```python
from build123d import *
from build123d.topology import SkipClean

# Parameters (mm, degrees)
BOSS_EXTRUDE1_DEPTH      = 10
SKETCH4_R                = 1.962636903
CUT_EXTRUDE2_DEPTH       = 10
SKETCH6_R                = 2.5
SKETCH6_R_2              = 1.962636903
BOSS_EXTRUDE2_DEPTH      = 3.333333333
BOSS_EXTRUDE3_START      = -3.333333333
SKETCH7_R                = 2.5
SKETCH7_R_2              = 1.962636903
BOSS_EXTRUDE3_DEPTH      = 3.333333333
SKETCH9_W                = 3.333333334
SKETCH9_H                = 5
CUT_EXTRUDE7_DEPTH       = 3
SKETCH10_W               = 3.333333334
SKETCH10_H               = 1.037363097
CUT_EXTRUDE8_DEPTH       = 37.201372358
BOSS_EXTRUDE4_DEPTH      = 1.5
BOSS_EXTRUDE4_DEPTH_BACK = 1.5
SKETCH12_R               = 2
BOSS_EXTRUDE9_DEPTH      = 1.5
BOSS_EXTRUDE9_DEPTH_BACK = 1.5
CUT_EXTRUDE9_DEPTH       = 40.05524944


with BuildPart() as part:
    # Sketch3 → Boss-Extrude1 (new body)
    with BuildSketch(Plane(origin=(0, 0, 0), x_dir=(0, 0, -1), z_dir=(1, 0, 0))):
        Polygon((30, 2.5), (31.962636903, 2.5), (31.97894003, 5), (30, 5), (0, 5), (0, 0), (30, 0), align=None)
    extrude(amount=BOSS_EXTRUDE1_DEPTH)

    # Sketch4 → Cut-Extrude2 (cut)
    with BuildSketch(Plane(origin=(0, 0, 0), x_dir=(0, 0, -1), z_dir=(1, 0, 0))):
        with Locations((31.962636903, 2.5)):
            Circle(SKETCH4_R)
    extrude(amount=CUT_EXTRUDE2_DEPTH, mode=Mode.SUBTRACT)

    # Sketch6 → Boss-Extrude2 (add)
    with BuildSketch(Plane.ZY):
        with Locations((-31.962636903, 2.5)):
            Circle(SKETCH6_R)
        with Locations((-31.962636903, 2.5)):
            Circle(SKETCH6_R_2, mode=Mode.SUBTRACT)
    extrude(amount=-BOSS_EXTRUDE2_DEPTH)

    # Sketch7 → Boss-Extrude3 (add)
    with BuildSketch(Plane(origin=(10, 0, 0), x_dir=(0, 0, -1), z_dir=(1, 0, 0)).offset(BOSS_EXTRUDE3_START)):
        with Locations((31.962636903, 2.5)):
            Circle(SKETCH7_R)
        with Locations((31.962636903, 2.5)):
            Circle(SKETCH7_R_2, mode=Mode.SUBTRACT)
    extrude(amount=BOSS_EXTRUDE3_DEPTH)

    # Sketch9 → Cut-Extrude7 (cut)
    with SkipClean():  # the faces are left unmerged after this step: merging them gives an invalid solid
        with BuildSketch(Plane(origin=(0, -0.208321197, -31.944975261), x_dir=(-1, 0, 0), z_dir=(0, -0.006521112201233067, -0.9999787373217788))):
            with Locations((-5, 2.708378785)):
                Rectangle(SKETCH9_W, SKETCH9_H)
        extrude(amount=-CUT_EXTRUDE7_DEPTH, mode=Mode.SUBTRACT)

    # Sketch10 → Cut-Extrude8 (cut, through all)
    with SkipClean():  # the faces are left unmerged after this step: merging them gives an invalid solid
        with BuildSketch(Plane(origin=(0, 0.208374354, -0.001358861), x_dir=(1, 0, 0), z_dir=(0, 0.9999787373217788, -0.00652111220123307))):
            with Locations((5, 29.464336059)):
                Rectangle(SKETCH10_W, SKETCH10_H)
        extrude(amount=-CUT_EXTRUDE8_DEPTH, mode=Mode.SUBTRACT)

    # Sketch12 → Boss-Extrude4 (add, two sides: drawn at the far end of the back side and taken through both)
    with SkipClean():  # the faces are left unmerged after this step: merging them gives an invalid solid
        with BuildSketch(Plane(origin=(5, 0, 0), x_dir=(0, 0, -1), z_dir=(1, 0, 0)).offset(-BOSS_EXTRUDE4_DEPTH_BACK)):
            with BuildLine():
                Line((-2.5, 5), (0, 5))
                Line((0, 5), (0, 2.5))
                ThreePointArc((0, 2.5), (-4.267766953, 0.732233047), (-2.5, 5))
            make_face()
            with Locations((-2.5, 2.5)):
                Circle(SKETCH12_R, mode=Mode.SUBTRACT)
        extrude(amount=BOSS_EXTRUDE4_DEPTH + BOSS_EXTRUDE4_DEPTH_BACK)

    # Sketch13 → Boss-Extrude9 (add, two sides: drawn at the far end of the back side and taken through both)
    with SkipClean():  # the faces are left unmerged after this step: merging them gives an invalid solid
        with BuildSketch(Plane(origin=(5, 0, 0), x_dir=(0, 0, -1), z_dir=(1, 0, 0)).offset(-BOSS_EXTRUDE9_DEPTH_BACK)):
            with BuildLine():
                Line((24.809137755, 5), (28, 5))
                Line((28, 5), (38, 5))
                Line((38, 5), (38, 6.25))
                Line((38, 6.25), (28, 6.25))
                add(Edge.make_bspline(
                    [(28, 6.25), (27.570139782, 6.25), (27.108034748, 5.787413316), (26.444737385, 5.323894947), (26.11400028, 5.04700236), (24.809137755, 5.04700236)],
                    knots=[0, 0, 0, 0, 0.435997525, 0.535997525, 1, 1, 1, 1], degree=3))
                Line((24.809137755, 5.04700236), (24.809137755, 5))
            make_face()
        extrude(amount=BOSS_EXTRUDE9_DEPTH + BOSS_EXTRUDE9_DEPTH_BACK)

    # Sketch14 → Cut-Extrude9 (cut, through all)
    with SkipClean():  # the faces are left unmerged after this step: merging them gives an invalid solid
        with BuildSketch(Plane(origin=(6.5, 0, 0), x_dir=(0, 0, -1), z_dir=(1, 0, 0))):
            Polygon((31.97894003, 5), (31.97894003, 5.19699687), (35.810977428, 5.19699687), (35.810977428, 6.25), (38, 6.25), (38, 5.19699687), (38, 5), align=None)
        extrude(amount=-CUT_EXTRUDE9_DEPTH, mode=Mode.SUBTRACT)


solid = part.part
```
Source: CAD feature listing. Evaluate the final solid. Frame: model axes, mm. A direction names the side the tool comes from. Round coordinates to 2 decimals unless told otherwise and drop trailing zeros. Order: outer loops, then holes, each group sorted by start corner. A loop starts at its lowest first (then second) coordinate and runs counter-clockwise, first axis right, second up. Notation, with made-up numbers: (40.5, 55.25) -> (93.5, 55.25) arc R25 ccw to (93.5, 78.25) -> close; hole circle Ø9 at (3, 12.25). An arc over 180 degrees is marked (long way). One line per item, written item: value. Start each with the question number.
Q1. Material intervals for probe 1 along Z at (x, y) = (2.4, 2.5); probe 2 along Y at (x, z) = (4.95, 2.5); probe 3 along Y at (x, z) = (9.5, -11.5), sorted ascending.
Q2. Section query C-C (y = 3). Return the cut outline in (x, z).
Q3. Section query D-D (z = -33). Return the cut outline in (x, y), plus the area to 3 significant figures.
Q4. Draft query along X for faces 1 (the flat face through (3.5, 6, -31)), 2 (the flat face through (5, 5, -30)), 3 (the flat face through (10, 3, -17)), 4 (the flat face through (5, 0, -15)). Return one class per face: pulls with the +X half, pulls with the -X half, needs draft (parallel to the pull), parting line crosses it, or undercut.
Q5. Section query B-B (z = 1). Return the cut outline in (x, y), plus the area to 3 significant figures.
Q6. Access query for faces 5 (the flat face through (6.5, 4, 0.8)), 6 (the flat face through (5, 5.197, -34)), 7 (the flat face through (6.5, 6, -31)), 8 (the flat face through (3.5, 4, 0.8)). Directions: +Z, -Z, +X, -X, +Y, -Y. A direction counts if a zero-diameter tool reaches every point of the face in a straight line with its end or side. Return the directions, or none.
Q7. Pin query (flat end, axial travel): pin 1 (1.5 mm diameter, centred on y = 1.5, z = 2.5, fed in from -X); pin 2 (1.5 mm diameter, centred on x = 5, z = -31, fed in from -Y); pin 3 (0.9 mm diameter, centred on x = 4.5, z = -34, fed in from -Y); pin 4 (1 mm diameter, centred on x = 4.5, z = -4, fed in from +Y). Return the tip coordinate at first contact, or that it passes through.
Findings below:
1. probe 1: -34.46 to -33.93, -30 to 0
1. probe 2: 0 to 0.5, 4.5 to 5
1. probe 3: 0 to 5
2. outline: (0, -34.41) -> (3.33, -34.41) -> (3.33, -33.86) -> (0, -33.86) -> close; (0, -30.06) -> (3.33, -30.06) -> (3.33, -28.97) -> (6.67, -28.97) -> (6.67, -30.06) -> (10, -30.06) -> (10, 0) -> (6.5, 0) -> (6.5, 0.56) -> (3.5, 0.56) -> (3.5, 0) -> (0, 0) -> close; (3.5, 4.44) -> (6.5, 4.44) -> (6.5, 4.95) -> (3.5, 4.95) -> close; (6.67, -34.41) -> (10, -34.41) -> (10, -33.86) -> (6.67, -33.86) -> close
3. outline: (0, 0.23) -> (3.33, 0.23) -> (3.33, 0.83) -> (0, 0.83) -> close; (0, 4.17) -> (3.33, 4.17) -> (3.33, 4.77) -> (0, 4.77) -> close; (3.5, 5.2) -> (6.5, 5.2) -> (6.5, 6.25) -> (3.5, 6.25) -> close; (6.67, 0.23) -> (10, 0.23) -> (10, 0.83) -> (6.67, 0.83) -> close; (6.67, 4.17) -> (10, 4.17) -> (10, 4.77) -> (6.67, 4.77) -> close
3. area: 11.3 mm²
4. face 1: pulls with the -X half
4. face 2: undercut
4. face 3: pulls with the +X half
4. face 4: needs draft
5. outline: (3.5, 0.5) -> (6.5, 0.5) -> (6.5, 1.18) -> (3.5, 1.18) -> close; (3.5, 3.82) -> (6.5, 3.82) -> (6.5, 5) -> (3.5, 5) -> close
5. area: 5.56 mm²
6. face 5: +Z, +X, +Y, -Y
6. face 6: -Z, +X, -X, -Y
6. face 7: +Z, -Z, +X, +Y
6. face 8: +Z, -X, +Y, -Y
7. pin 1: through
7. pin 2: y = 5
7. pin 3: y = 5.2
7. pin 4: y = 5
